```python
from build123d import *

# Parameters (mm, degrees)
BOSS_EXTRUDE6_DEPTH = 0.17
CUT_EXTRUDE4_DEPTH  = 62.727456614


with BuildPart() as part:
    # Sketch20 → Boss-Extrude6 (new body)
    with BuildSketch(Plane.XY):
        with BuildLine():
            Line((-12.5, 60), (4.5, 60))
            ThreePointArc((4.5, 60), (11.571067812, 57.071067812), (14.5, 50))
            Line((14.5, 50), (14.5, -58))
            ThreePointArc((14.5, -58), (13.914213562, -59.414213562), (12.5, -60))
            Line((12.5, -60), (-12.5, -60))
            ThreePointArc((-12.5, -60), (-13.914213562, -59.414213562), (-14.5, -58))
            Line((-14.5, -58), (-14.5, 58))
            ThreePointArc((-14.5, 58), (-13.914213562, 59.414213562), (-12.5, 60))
        make_face()
    extrude(amount=BOSS_EXTRUDE6_DEPTH)

    # Sketch14 → Cut-Extrude4 (cut, through all)
    with BuildSketch(Plane.XY.offset(0.17)):
        with BuildLine():
            Line((-1.9, -29), (1.9, -29))
            Line((1.9, -29), (8.375, -42.75))
            add(Edge.make_bspline(
                [(8.375, -42.75), (8.614001568, -43.20601542), (8.749703343, -43.736930638), (8.75, -44.3)],
                knots=[2, 2, 2, 2, 3, 3, 3, 3], degree=3))
            add(Edge.make_bspline(
                [(8.75, -44.3), (8.75059415, -45.427724457), (8.211440188, -46.416320927), (7.4, -46.97314145)],
                knots=[3, 3, 3, 3, 3.998304655, 3.998304655, 3.998304655, 3.998304655], degree=3))
            Line((7.4, -46.97314145), (4.925, -48.85))
            add(Edge.make_bspline(
                [(4.925, -48.85), (3.956162506, -45.631727685), (2.146734918, -43.400643505), (0, -43.4)],
                knots=[5.0019278, 5.0019278, 5.0019278, 5.0019278, 5.999902224, 5.999902224, 5.999902224, 5.999902224], degree=3))
            add(Edge.make_bspline(
                [(-4.925, -48.85), (-3.956162506, -45.631727685), (-2.146734918, -43.400643505), (0, -43.4)],
                knots=[5.0019278, 5.0019278, 5.0019278, 5.0019278, 5.999902224, 5.999902224, 5.999902224, 5.999902224], degree=3))
            Line((-4.925, -48.85), (-7.4, -46.97314145))
            add(Edge.make_bspline(
                [(-8.75, -44.3), (-8.75059415, -45.427724457), (-8.211440188, -46.416320927), (-7.4, -46.97314145)],
                knots=[3, 3, 3, 3, 3.998304655, 3.998304655, 3.998304655, 3.998304655], degree=3))
            add(Edge.make_bspline(
                [(-8.375, -42.75), (-8.614001568, -43.20601542), (-8.749703343, -43.736930638), (-8.75, -44.3)],
                knots=[2, 2, 2, 2, 3, 3, 3, 3], degree=3))
            Line((-8.375, -42.75), (-1.9, -29))
        make_face()
    extrude(amount=-CUT_EXTRUDE4_DEPTH, mode=Mode.SUBTRACT)


solid = part.part
```
Design review of the part built by this model. Coordinates are the model's own, in mm. Round coordinates to 2 decimals unless told otherwise and drop trailing zeros. Write each loop counter-clockwise with the first axis right and the second up, starting at its lowest first coordinate (ties: lowest second). Pieces come first, ordered by that corner, then holes. Notation, with made-up numbers: (-36, 25) -> (17, 25) arc R16 ccw to (17, 34) -> close; hole circle Ø6 at (27.25, 69.25). An arc over 180 degrees is marked (long way). Write item = value, one per line. Start each with the question number.
1) Take a section at C-C, the plane x = 11. State the section outline as (y, z) points.
2) Wall thickness on probe 1 along X at (y, z) = (-45.5, 0.1); probe 2 along Y at (x, z) = (0.75, 0.1); probe 3 along Y at (x, z) = (10.5, 0.1): over which ranges is each line inside the solid? List them lowest first. Write a range as from..to.
3) Take a section at B-B, the plane x = 6. State the section outline as (y, z) points.
4) Clearance check with a flat-ended pin moving along its axis: pin 1 (3 mm diameter, centred on x = -2.5, y = 39.5, fed in from -Z). State where the tip first meets the part, or that it passes through.
5) Take a section at A-A, the plane y = -38.5. State the section outline as (x, z) points, plus the area to 3 significant figures.
Results list:
q1.outline = (-60, 0) -> (57.6, 0) -> (57.6, 0.17) -> (-60, 0.17) -> close
q2.probe_1 = -14.5..-8.54, -3.36..3.36, 8.54..14.5
q2.probe_2 = -60..-43.49, -29..60
q2.probe_3 = -60..58
q3.outline = (-60, 0) -> (-48.03, 0) -> (-48.03, 0.17) -> (-60, 0.17) -> close; (-37.71, 0) -> (59.89, 0) -> (59.89, 0.17) -> (-37.71, 0.17) -> close
q4.pin_1 = 0
q5.outline = (-14.5, 0) -> (-6.37, 0) -> (-6.37, 0.17) -> (-14.5, 0.17) -> close; (6.37, 0) -> (14.5, 0) -> (14.5, 0.17) -> (6.37, 0.17) -> close
q5.area = 2.76 mm²
